Can you work these out from the model? Positions are in its coordinate system, mm. A direction names the side the tool comes from. Give positions to 0.01 mm unless a question says otherwise; leave off trailing zeros. Write each loop counter-clockwise with the first axis right and the second up, starting at its lowest first coordinate (ties: lowest second). Pieces come first, ordered by that corner, then holes. Notation, with made-up numbers: M 45,69 L 72,69 A18 cw 72,93 Z; hole C 22.25,72 d3. An arc over 180 degrees is marked long. Use CSV: the item, a comma, the result in double quotes. Start each with the question number.
Autodesk Inventor part; units mm, degrees
ref_plane "Work Plane1" through (0, 0, -23.75) normal (0, 0, 1) x (1, 0, 0)
ref_plane "YZ Plane" through (0, 0, 0) normal (1, 0, 0) x (0, 1, 0)
ref_plane "XZ Plane" through (0, 0, 0) normal (0, 1, 0) x (-1, 0, 0)
sketch "Sketch1" plane through (0, 0, 0) normal (0, 1, 0) x (-1, 0, 0)
  line L0 (0, 0) -> (26, 0)
  line L1 (26, 0) -> (26, -47.5)
  line L2 (26, -47.5) -> (0, -47.5)
  line L3 (0, -47.5) -> (0, 0)
  dimension "d0" = 26
  dimension "d1" = 47.5
extrude "Extrusion1" add sketch "Sketch1" along normal blind 14
sketch "Sketch2" plane through (0, 14, 0) normal (0, 1, 0) x (1, 0, 0)
  line L0 (-26, 0) -> (0, 0)
  line L1 (-13, 0) -> (-13, -8.75)
  line L2 (-13, -8.75) -> (-13, 0) construction
  line L3 (-11.25, -8.75) -> (-11.25, 0)
  line L4 (-14.75, 0) -> (-14.75, -8.75)
  arc A0 (-14.75, -8.75) -> (-11.25, -8.75) centre (-13, -8.75) ccw
  arc A1 (-11.25, 0) -> (-14.75, 0) centre (-13, 0) ccw
  line L5 (-14.75, -8.75) -> (-17.5, -8.75)
  line L6 (-11.25, -8.75) -> (-8.5, -8.75)
  line L7 (-11.25, -8.75) -> (-14.75, -8.75)
  line L8 (-26, 0) -> (-19.75, 0)
  line L9 (-19.75, 0) -> (-17.5, -8.75)
  line L10 (0, 0) -> (-6.25, 0)
  line L11 (-6.25, 0) -> (-8.5, -8.75)
  point P0 (-13, -4.375)
  dimension "d4" = 8.75
  dimension "d5" = 3.5
  dimension "d6" = 2.75
  dimension "d7" = 2.75
  dimension "d8" = 6.25
  dimension "d9" = 6.25
extrude "Extrusion2" add sketch "Sketch2" against normal blind 3.5 contours L0 L4 L5 L9 | L0 L11 L6 L3
ref_plane "Work Plane1" through (0, 0, -23.75) normal (0, 0, 1) x (1, 0, 0)
mirror "Mirror1" about plane through (0, 0, -23.75) normal (0, 0, 1) of "Extrusion2"
sketch "Sketch4" plane through (0, 0, 0) normal (1, 0, 0) x (0, 0, -1)
  line L0 (0, 0) -> (0, 14)
  line L1 (0, 0) -> (0, 5)
  line L2 (0, 5) -> (5, 5)
  circle A0 centre (5, 5) radius 1.25
  circle A1 centre (2.5, 5) radius 1.25
  line L3 (0, 0) -> (47.5, 0)
  line L4 (47.5, 0) -> (47.5, 5)
  line L5 (47.5, 0) -> (47.5, 14)
  line L6 (47.5, 5) -> (42.5, 5)
  circle A2 centre (42.5, 5) radius 1.25
  circle A3 centre (45, 5) radius 1.25
  point P0 (43.75, 5)
  point P1 (3.75, 5)
  dimension "d13" = 5
  dimension "d14" = 5
  dimension "d15" = 2.5
  dimension "d16" = 2.5
  dimension "d17" = 5
  dimension "d18" = 5
  dimension "d19" = 2.5
  dimension "d20" = 2.5
extrude "Extrusion3" add sketch "Sketch4" along normal blind 7.5
properties part number "12_24_5VUSBConverter"
(1) I want a section at C-C (y = 12.5). Write out the boundary of the cut face in (x, z), and give its area (3 significant figures).
(2) Which directions (+Z, -Z, +X, -X, +Y, -Y) give clear straight access to the entire face, cutting with the end or side of a thin tool? Please do faces 4 (the face through (-17, 10.5, -52)), 5 (the face through (-11.25, 12, 4)), 6 (the face through (-9, 10.5, 4)).
(3) Will these pins go through, and if not, where does the flat tip stop? pin 1 Ø2.5 at (x, z) = (-8.5, 4) entering from -Y; pin 2 Ø1 at (y, z) = (12.5, 2.5) entering from -X; pin 3 Ø4 at (x, y) = (3, 2.5) entering from +Z.
(4) Thinking about a two-plate mould opening in Z: for faces 1 (the face through (3.7, 5.76, -41.51)), 2 (the face through (7.5, 5, -42)), 3 (the face through (-16, 12, 8.75)), which applies, released by +Z, released by -Z, zero draft, split by the parting line, or undercut?
(5) I want a section at B-B (x = -9.5). Write out the boundary of the cut face in (y, z), and give its area (3 significant figures).
(6) I want a section at A-A (z = -5). Write out the boundary of the cut face in (x, y).
(7) Please list where these lines run through material, in increasing order: L1, parallel to X at y = 13.75, z = -39; L2, parallel to X at y = 13.5, z = -52; L3, parallel to Y at x = -18, z = -49. Write a range as [from, to].
(8) I want a section at D-D (z = -48.5). Write out the boundary of the cut face in (x, y), and give its area (3 significant figures).
Geometry results:
1,outline,"M -26,-47.5 L -19.75,-47.5 L -17.5,-56.25 L -14.75,-56.25 L -14.75,-47.5 L -11.25,-47.5 L -11.25,-56.25 L -8.5,-56.25 L -6.25,-47.5 L 0,-47.5 L 0,0 L -6.25,0 L -8.5,8.75 L -11.25,8.75 L -11.25,0 L -14.75,0 L -14.75,8.75 L -17.5,8.75 L -19.75,0 L -26,0 Z"
1,area,"1,370 mm2"
2,face 4,"-Z, +X, -X, -Y"
2,face 5,"+Z, +Y, -Y"
2,face 6,"+Z, +X, -X, -Y"
3,pin 1,"stops at y = 10.5"
3,pin 2,"stops at x = -19.24"
3,pin 3,"stops at z = -1.35"
4,face 1,"undercut"
4,face 2,"zero draft"
4,face 3,"released by +Z"
5,outline,"M 0,-47.5 L 10.5,-47.5 L 10.5,-56.25 L 14,-56.25 L 14,8.75 L 10.5,8.75 L 10.5,0 L 0,0 Z"
5,area,"726 mm2"
6,outline,"M -26,0 L 0,0 L 0,3.75 L 7.5,3.75 L 7.5,6.25 L 0,6.25 L 0,14 L -26,14 Z"
7,L1,"x = [-26, 0]"
7,L2,"x = [-18.59, -14.75], [-11.25, -7.41]"
7,L3,"y = [10.5, 14]"
8,outline,"M -19.49,10.5 L -14.75,10.5 L -14.75,14 L -19.49,14 Z; M -11.25,10.5 L -6.51,10.5 L -6.51,14 L -11.25,14 Z"
8,area,"33.2 mm2"
